```python
from build123d import *

# Parameters (mm, degrees)
SKETCH1_R           = 8.88
SKETCH1_R_2         = 1.6
BOSS_EXTRUDE1_DEPTH = 6.5
BOSS_EXTRUDE2_START = 6.5
SKETCH1_3_R         = 10.38
SKETCH1_3_R_2       = 1.6
BOSS_EXTRUDE2_DEPTH = 1.5
SKETCH2_R           = 2.35
SKETCH2_R_2         = 2.1
CUT_EXTRUDE1_DEPTH  = 1.2
SKETCH2_2_R         = 2.1
CUT_EXTRUDE2_DEPTH  = 5
SKETCH3_R           = 0.925
CUT_EXTRUDE3_DEPTH  = 3


with BuildPart() as part:
    # Sketch1 → Boss-Extrude1 (new body)
    with BuildSketch(Plane(origin=(0, 0, 0), x_dir=(1, 0, 0), z_dir=(0, 1, 0))):
        with Locations(Location((0, 0, 0), (0, 0, 90))):
            Circle(SKETCH1_R)
        with Locations(Location((0, 0, 0), (0, 0, 90))):
            Circle(SKETCH1_R_2, mode=Mode.SUBTRACT)
    extrude(amount=BOSS_EXTRUDE1_DEPTH)

    # Sketch1<3> → Boss-Extrude2 (add)
    with BuildSketch(Plane(origin=(0, 0, 0), x_dir=(1, 0, 0), z_dir=(0, 1, 0)).offset(BOSS_EXTRUDE2_START)):
        with Locations(Location((0, 0, 0), (0, 0, 270))):
            Circle(SKETCH1_3_R)
        with Locations(Location((0, 0, 0), (0, 0, 90))):
            Circle(SKETCH1_3_R_2, mode=Mode.SUBTRACT)
    extrude(amount=BOSS_EXTRUDE2_DEPTH)

    # Sketch2 → Cut-Extrude1 (cut)
    with BuildSketch(Plane(origin=(0, 0, -8.88), x_dir=(-1, 0, 0), z_dir=(0, 0, -1))):
        with Locations((0, 2.75)):
            Circle(SKETCH2_R)
        with Locations((0, 2.75)):
            Circle(SKETCH2_R_2, mode=Mode.SUBTRACT)
    extrude(amount=-CUT_EXTRUDE1_DEPTH, mode=Mode.SUBTRACT)

    # Sketch2<2> → Cut-Extrude2 (cut)
    with BuildSketch(Plane(origin=(0, 0, -8.88), x_dir=(-1, 0, 0), z_dir=(0, 0, -1))):
        with Locations((0, 2.75)):
            Circle(SKETCH2_2_R)
    extrude(amount=-CUT_EXTRUDE2_DEPTH, mode=Mode.SUBTRACT)

    # Sketch3 → Cut-Extrude3 (cut)
    with BuildSketch(Plane(origin=(0, 8, 0), x_dir=(1, 0, 0), z_dir=(0, 1, 0))):
        with Locations(Location((-5.218448045, 5.218448045, 0), (0, 0, 270))):
            Circle(SKETCH3_R)
        with Locations(Location((-5.218448045, -5.218448045, 0), (0, 0, 270))):
            Circle(SKETCH3_R)
        with Locations(Location((5.218448045, -5.218448045, 0), (0, 0, 270))):
            Circle(SKETCH3_R)
        with Locations(Location((5.218448045, 5.218448045, 0), (0, 0, 270))):
            Circle(SKETCH3_R)
    extrude(amount=-CUT_EXTRUDE3_DEPTH, mode=Mode.SUBTRACT)


solid = part.part
```
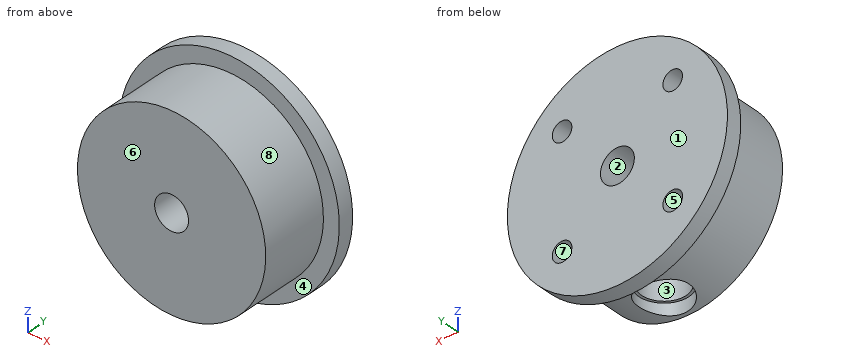
CAD build for the part. Positions are in the model's coordinates, mm. Face numbers are marked on the shaded views. A direction names the side the tool comes from. Give positions to 0.01 mm unless a question says otherwise; leave off trailing zeros. Loops run counter-clockwise (first coordinate to the right, second up) from the corner with the lowest first, then second, coordinate; pieces in that order, holes last. Notation, with made-up numbers: (-8, 75) -> (20, 75) arc R29 ccw to (20, 101) -> close; hole circle Ø2 at (79, 24.5). An arc over 180 degrees is marked (long way). Use a Markdown table: item, result.
1. Flat gauge pins, fed straight in: pin 1 (3 mm diameter, centred on y = 6, z = -3, fed in from +X); pin 2 (4 mm diameter, centred on x = 1, y = 2, fed in from -Z); pin 3 (1 mm diameter, centred on x = -3, y = 7, fed in from +Z). Where does each tip first touch, or does it go through?
Check result:
| item | result |
|---|---|
| pin 1 | stops at x = 10.26 |
| pin 2 | stops at z = -8.88 |
| pin 3 | stops at z = 10.07 |
2. Slice it at A-A (x = 0). List the corners of the cut face in (y, z).
Check result:
| item | result |
|---|---|
| outline | (0, -8.88) -> (0.4, -8.88) -> (0.4, -7.68) -> (0.65, -7.68) -> (0.65, -3.88) -> (4.85, -3.88) -> (4.85, -7.68) -> (5.1, -7.68) -> (5.1, -8.88) -> (6.5, -8.88) -> (6.5, -10.38) -> (8, -10.38) -> (8, -1.6) -> (0, -1.6) -> close; (0, 1.6) -> (8, 1.6) -> (8, 10.38) -> (6.5, 10.38) -> (6.5, 8.88) -> (0, 8.88) -> close |
3. Slice it at B-B (z = 0). List the corners of the cut face in (x, y), plus the area to 3 significant figures.
Check result:
| item | result |
|---|---|
| outline | (-10.38, 6.5) -> (-8.88, 6.5) -> (-8.88, 0) -> (-1.6, 0) -> (-1.6, 8) -> (-10.38, 8) -> close; (1.6, 0) -> (8.88, 0) -> (8.88, 6.5) -> (10.38, 6.5) -> (10.38, 8) -> (1.6, 8) -> close |
| area | 121 mm^2 |
4. Slice it at D-D (y = 2.75). List the corners of the cut face in (x, z), plus the area to 3 significant figures.
Check result:
| item | result |
|---|---|
| outline | (-2.35, -8.56) -> (-2.35, -7.68) -> (-2.1, -7.68) -> (-2.1, -3.88) -> (2.1, -3.88) -> (2.1, -7.68) -> (2.35, -7.68) -> (2.35, -8.56) arc R8.88 ccw (long way) to start; hole circle Ø3.2 at (0, 0) |
| area | 219 mm^2 |
5. Slice it at C-C (z = -7). List the corners of the cut face in (x, y).
Check result:
| item | result |
|---|---|
| outline | (-7.66, 6.5) -> (-5.46, 6.5) -> (-5.46, 0) -> (5.46, 0) -> (5.46, 6.5) -> (7.66, 6.5) -> (7.66, 8) -> (-7.66, 8) -> close; hole circle Ø4.2 at (0, 2.75) |
6. Wall check: L1, parallel to X at y = 7, z = -5.25; L2, parallel to X at y = 5.5, z = -5; L3, parallel to Y at x = 1, z = 9.5. Give the ranges that are in metal, low to high. Write a range as [from, to].
Check result:
| item | result |
|---|---|
| L1 | x = [-8.95, -6.14], [-4.29, 4.29], [6.14, 8.95] |
| L2 | x = [-7.34, -6.12], [-4.32, 4.32], [6.12, 7.34] |
| L3 | y = [6.5, 8] |
7. Mould opens along Z. For the marked faces 6, 7 and 8 say: pulls with the +Z half, pulls with the -Z half, needs draft (parallel to the pull), parting line crosses it, or undercut.
Check result:
| item | result |
|---|---|
| face 6 | needs draft |
| face 7 | undercut |
| face 8 | parting line crosses it |
8. Which spindle directions (+Z, -Z, +X, -X, +Y, -Y) get a long thin tool onto all of the face, cutting with end or side? Do the marked faces 1, 2, 3, 4 and 5. Say none if no direction does.
Check result:
| item | result |
|---|---|
| face 1 | +Z, -Z, +X, -X, +Y |
| face 2 | +Y, -Y |
| face 3 | -Z |
| face 4 | -Y |
| face 5 | +Y |
